from build123d import *

# Parameters (mm, degrees)
F0_R     = 28.575
F1_DEPTH = 7.9375


with BuildPart() as f1:
    # F0 (on Top) → F1 (new body)
    with BuildSketch(Plane.XY):
        Circle(F0_R)
        with BuildLine():
            ThreePointArc((3.96875, 15.370903), (11.22532, 11.22532), (15.370903, 3.96875))
            Line((15.370903, 3.96875), (21.720903, 3.96875))
            Line((21.720903, 3.96875), (21.720903, -3.96875))
            Line((21.720903, -3.96875), (15.370903, -3.96875))
            ThreePointArc((15.370903, -3.96875), (11.22532, -11.22532), (3.96875, -15.370903))
            Line((3.96875, -15.370903), (3.96875, -21.720903))
            Line((3.96875, -21.720903), (-3.96875, -21.720903))
            Line((-3.96875, -21.720903), (-3.96875, -15.370903))
            ThreePointArc((-3.96875, -15.370903), (-11.22532, -11.22532), (-15.370903, -3.96875))
            Line((-15.370903, -3.96875), (-21.720903, -3.96875))
            Line((-21.720903, -3.96875), (-21.720903, 3.96875))
            Line((-21.720903, 3.96875), (-15.370903, 3.96875))
            ThreePointArc((-15.370903, 3.96875), (-11.22532, 11.22532), (-3.96875, 15.370903))
            Line((-3.96875, 15.370903), (-3.96875, 21.720903))
            Line((-3.96875, 21.720903), (3.96875, 21.720903))
            Line((3.96875, 21.720903), (3.96875, 15.370903))
        make_face(mode=Mode.SUBTRACT)
    extrude(amount=F1_DEPTH)


solid = f1.part
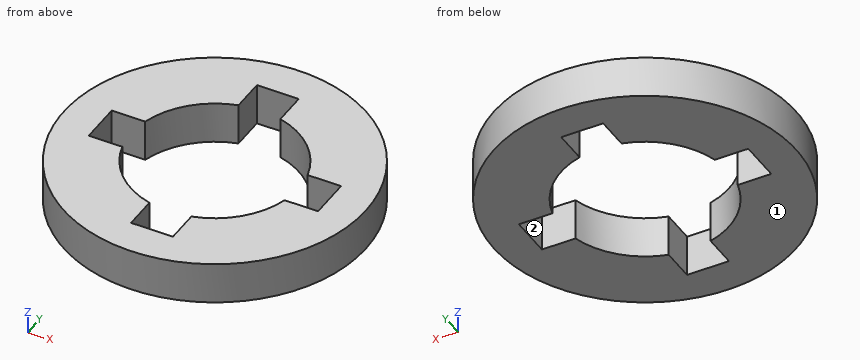
Geometry check sheet. Reference: the model listing, model coordinates, mm. Face numbers are marked on the shaded views. A direction names the side the tool comes from. Give positions to 0.01 mm unless a question says otherwise; leave off trailing zeros. Order: outer loops, then holes, each group sorted by start corner. A loop starts at its lowest first (then second) coordinate and runs counter-clockwise, first axis right, second up.
1) Material ranges on probe 1 along X at (y, z) = (-0.5, 3.75); probe 2 along X at (y, z) = (2.5, 5); probe 3 along Y at (x, z) = (12, 2), recorded low to high.
Results are:
probe 1: x = -28.57 to -21.72, 21.72 to 28.57
probe 2: x = -28.47 to -21.72, 21.72 to 28.47
probe 3: y = -25.93 to -10.39, 10.39 to 25.93
2) Cross-section at A-A (x = 0). Record the boundary of the cut face in (y, z) (1 decimal).
Results are:
outline: (-28.6, 0) - (-21.7, 0) - (-21.7, 7.9) - (-28.6, 7.9) - close; (21.7, 0) - (28.6, 0) - (28.6, 7.9) - (21.7, 7.9) - close
3) Tool access check on the marked faces 1 and 2. Record the directions out of +Z, -Z, +X, -X, +Y, -Y that give a thin tool (end or side, any length) a straight path to the whole face; none if there is none.
Results are:
face 1: -Z, +X, -X, +Y, -Y
face 2: +Z, -Z
4) Gauge pin test, flat end, axial feed: pin 1 (2.5 mm diameter, centred on x = -0.5, z = 6, fed in from -Y) (3 decimals). Record the tip position at first contact, or that the pin passes through.
Results are:
pin 1: stops at y = -28.575
5) Cross-section at D-D (y = -25). Record the boundary of the cut face in (x, z), then the cut area to 3 significant figures.
Results are:
outline: (-13.84, 0) - (13.84, 0) - (13.84, 7.94) - (-13.84, 7.94) - close
area: 220 mm2
6) Cross-section at C-C (z = 5.25). Record the boundary of the cut face in (x, y) (3 decimals), then the cut area to 3 significant figures.
Results are:
outline: circle Ø57.15 at (0, 0); hole (-21.721, -3.969) - (-15.371, -3.969) arc R15.875 ccw to (-3.969, -15.371) - (-3.969, -21.721) - (3.969, -21.721) - (3.969, -15.371) arc R15.875 ccw to (15.371, -3.969) - (21.721, -3.969) - (21.721, 3.969) - (15.371, 3.969) arc R15.875 ccw to (3.969, 15.371) - (3.969, 21.721) - (-3.969, 21.721) - (-3.969, 15.371) arc R15.875 ccw to (-15.371, 3.969) - (-21.721, 3.969) - close
area: 1,580 mm2
